```python
from build123d import *

# Parameters (mm, degrees)
F0_W     = 1524
F0_H     = 914.4
F1_DEPTH = 838.2
F2_W     = 403.0548334122
F2_H     = 305.4204545915
F3_DEPTH = 88.392
F4_W     = 90.1145935059
F4_H     = 56.3738569617
F5_DEPTH = 179.832
F6_W     = 90.1145935059
F6_H     = 28.3284043617
F7_DEPTH = 60.96


with BuildPart() as f1:
    # F0 (on Top) → F1 (new body)
    with BuildSketch(Plane.XY):
        with Locations((-449.5147587423, 11.9446208701)):
            Rectangle(F0_W, F0_H)
    extrude(amount=F1_DEPTH)

    # F2 (on face) → F3 (cut)
    with BuildSketch(Plane.XY.offset(838.2)):
        with Locations((-939.5418763161, -176.386596635)):
            Rectangle(F2_W, F2_H)
    extrude(amount=-F3_DEPTH, mode=Mode.SUBTRACT)

    # F4 (on face) → F5 (join)
    with BuildSketch(Plane.XY.offset(838.2)):
        with Locations((-942.1632885933, 4.5105591416)):
            Rectangle(F4_W, F4_H)
    extrude(amount=F5_DEPTH)

    # F6 (on face) → F7 (join)
    with BuildSketch(Plane.XZ.offset(23.6763693392)):
        with Locations((-942.1632885933, 1003.8677978191)):
            Rectangle(F6_W, F6_H)
    extrude(amount=F7_DEPTH)


solid = f1.part
```
Read the model definition and answer for the solid it produces. Units are mm, in the model's axes. A direction names the side the tool comes from. Round coordinates to 2 decimals unless told otherwise and drop trailing zeros. Write each loop counter-clockwise with the first axis right and the second up, starting at its lowest first coordinate (ties: lowest second). Pieces come first, ordered by that corner, then holes. Notation, with made-up numbers: (35, 75.25) - (51, 75.25) arc R16 cw to (51, 80.25) - close; hole circle Ø1 at (-23.75, 50.5). An arc over 180 degrees is marked (long way). Use CSV: the item, a comma, the result in double quotes.
Q1. Find section C-C, the plane z = 913. Write down the section's boundary in (x, y), then the cut area to 3 significant figures.
Values:
outline,"(-987.22, -23.68) - (-897.11, -23.68) - (-897.11, 32.7) - (-987.22, 32.7) - close"
area,"5,080 mm²"
Q2. Each of these flat-tipped pins is pushed along its axis until it touches: pin 1 Ø14 at (x, z) = (-926, 1000.5) entering from -Y; pin 2 Ø8 at (x, y) = (-244, 295.5) entering from +Z. Where does it stop, or does it pass through?
Values:
pin 1,"stops at y = -84.64"
pin 2,"stops at z = 838.2"
Q3. Determine the mould class of faces 5 (the flat face through (-943, 32.697, 927)), 6 (the flat face through (-942, -23.676, 845)), 7 (the flat face through (312.485, 6, 413)) for opening direction Y: +Y half, -Y half, draft (parallel to the pull), parting line (faces both ways), or undercut.
Values:
face 5,"+Y half"
face 6,"undercut"
face 7,"draft"
Q4. Find section D-D, the plane y = 53. Write down the section's boundary in (x, z), then the cut area to 3 significant figures.
Values:
outline,"(-1211.51, 0) - (312.49, 0) - (312.49, 838.2) - (-1211.51, 838.2) - close"
area,"1,280,000 mm²"
Q5. Find section B-B, the plane y = -199.5. Write down the section's boundary in (x, z).
Values:
outline,"(-1211.51, 0) - (312.49, 0) - (312.49, 838.2) - (-738.01, 838.2) - (-738.01, 749.81) - (-1141.07, 749.81) - (-1141.07, 838.2) - (-1211.51, 838.2) - close"
Q6. Find section A-A, the plane x = -842.5. Write down the section's boundary in (y, z).
Values:
outline,"(-445.26, 0) - (469.14, 0) - (469.14, 838.2) - (-23.68, 838.2) - (-23.68, 749.81) - (-329.1, 749.81) - (-329.1, 838.2) - (-445.26, 838.2) - close"
Q7. A tool of negligible diameter and unlimited length cuts with its end or side. For faces 1 (the flat face through (-1141.069, -179, 795)), 2 (the flat face through (-897.106, 1, 927)), 3 (the flat face through (-987.221, 1, 927)), 4 (the flat face through (-943, -54, 989.704)), from which of +Z, -Z, +X, -X, +Y, -Y can it reach the whole face along a straight path? Write none if from no direction.
Values:
face 1,"+Z"
face 2,"+Z, +X, +Y, -Y"
face 3,"+Z, -X, +Y, -Y"
face 4,"+X, -X, -Y"
Q8. Straight lines are drawn through the part: line 1 along X through (y, z) = (-250, 829.5); line 2 along Z through (x, y) = (-518, -15.5); line 3 along Z through (x, y) = (-860.5, -107.5). For each, find the intervals that lie inside material, in ascending order.
Values:
line 1,"x = -1211.51 to -1141.07, -738.01 to 312.49"
line 2,"z = 0 to 838.2"
line 3,"z = 0 to 749.81"
